Read the model definition and answer for the solid it produces. Units are mm, in the model's axes. A direction names the side the tool comes from. Give positions to 0.01 mm unless a question says otherwise; leave off trailing zeros. Write each loop counter-clockwise with the first axis right and the second up, starting at its lowest first coordinate (ties: lowest second). Pieces come first, ordered by that corner, then holes. Notation, with made-up numbers: M -20,-30 L -4,-30 A15 cw -4,-14 Z; hole C 51,-10 d6. An arc over 180 degrees is marked long. Use a Markdown table: item, result. Add a question column.
Item 1: The mould has two halves that part along X. Classify faces 1 (the flat face through (60, -77.788, 0)), 2 (the flat face through (-69.85, -109, 0)), 3 (the cylindrical face through (-37.26, -0.72, 9.57)): pulls with the +X half, pulls with the -X half, needs draft (parallel to the pull), parting line crosses it, or undercut.
Item 2: For faces 4 (the cylindrical face through (0.943, 42.852, 0.178)), 5 (the flat face through (0, 28, 6.35)), 6 (the flat face through (-42.862, -35, 0)), 7 (the cylindrical face through (0.73, 28.45, 0.55)), 8 (the cylindrical face through (31.201, -103.976, -9.569)), determine the directions among +Z, -Z, +X, -X, +Y, -Y from which every point of the face is accessible in a straight line to the end or side of a thin tool.
Item 3: A cutting plane is placed at C-C on x = 0. Count the separate pieces of the cut face and the enclosed holes in it, then the cut area to 3 significant figures.
Item 4: Given P1, Ø8, axis at y = -21.5, z = -3, coming from the +X side; P2, Ø4.5, axis at x = 22.5, y = -76.5, coming from the +Z side; P3, Ø5, axis at x = 36.5, z = 1, coming from the +Y side, each flat-ended and moving along its own axis, determine where each tip first touches the part or whether it passes through.
Item 5: A cutting plane is placed at A-A on x = -57.15. Determine the outline of the cut face in (y, z), then the cut area to 3 significant figures.
Item 6: Consider probe 1 along X at (y, z) = (0, 3); probe 2 along X at (y, z) = (0, 9.75); probe 3 along X at (y, z) = (-31.75, -2.25). Determine where each line is inside the solid, lowest interval first. Write a range as [from, to].
Item 7: A cutting plane is placed at B-B on y = -7.5. Determine the outline of the cut face in (x, z).
from build123d import *

# Parameters (mm, degrees)
BOLT_CIRCLE_R                                     = 12.7
BOLT_CIRCLE_R_2                                   = 6.35
BASE_DEPTH                                        = 12.7
STRUCTURE_TUBE_CONNECTION_COUNTERBORE_D           = 6.7564
STRUCTURE_TUBE_CONNECTION_COUNTERBORE_CBORE_D     = 11.1125
STRUCTURE_TUBE_CONNECTION_COUNTERBORE_CBORE_DEPTH = 6.35
STRUCTURE_TUBE_CONNECTION_COUNTERBORE_PA_COUNT    = 4
SPINDLE_CONNECTION_COUNTERBORE_D                  = 6.7564
SPINDLE_CONNECTION_COUNTERBORE_CBORE_D            = 11.1125
SPINDLE_CONNECTION_COUNTERBORE_CBORE_DEPTH        = 6.35
SPINDLE_CONNECTION_COUNTERBORE_PATTERN_COUNT      = 4
SKETCH16_R                                        = 36.5125
STRUCTURE_TUBE_MOUNTING_POCKET_DEPTH              = 6.35
SKETCH17_R                                        = 36.5125
SPINDLE_MOUNTING_POCKET_DEPTH                     = 7.62
SKETCH18_R                                        = 9.525
LEAD_SCREW_THROUGH_HOLE_DEPTH                     = 9.525
SKETCH20_R                                        = 7.9375
RAIL_MOUNTING_PILOT_HOLES_DEPTH                   = 166.290695159
SKETCH27_R                                        = 2.38125
ALIGNMENT_FEATURES_DEPTH                          = 6.35
GENERIC_ROUNDING_FILLET_R                         = 6.35


with BuildPart() as part:
    # Bolt circle → Base (new, symmetric)
    with BuildSketch(Plane.XY):
        with BuildLine():
            Line((-42.8625, 0), (-42.8625, -77.7875))
            Line((-42.8625, -77.7875), (-69.85, -77.7875))
            Line((-69.85, -77.7875), (-69.85, -147.6375))
            Line((-69.85, -147.6375), (69.85, -147.6375))
            Line((69.85, -147.6375), (69.85, -77.7875))
            Line((69.85, -77.7875), (42.8625, -77.7875))
            Line((42.8625, -77.7875), (42.8625, 0))
            ThreePointArc((42.8625, 0), (0, 42.8625), (-42.8625, 0))
        make_face()
        Circle(BOLT_CIRCLE_R, mode=Mode.SUBTRACT)
        with Locations((0, -98.425)):
            Circle(BOLT_CIRCLE_R_2, mode=Mode.SUBTRACT)
    extrude(amount=BASE_DEPTH, both=True)

    # Structure tube connection counterbore (through all)
    with Locations(Plane(origin=(0, 0, -12.7), x_dir=(-1, 0, 0), z_dir=(0, 0, -1))):
        with Locations((0, -67.46875)):
            structure_tube_connection_counterbore = CounterBoreHole(STRUCTURE_TUBE_CONNECTION_COUNTERBORE_D / 2, STRUCTURE_TUBE_CONNECTION_COUNTERBORE_CBORE_D / 2, STRUCTURE_TUBE_CONNECTION_COUNTERBORE_CBORE_DEPTH)

    # Structure tube connection counterbore pa: Structure tube connection counterbore ×4 about axis
    structure_tube_connection_counterbore_pa_axis = Axis((0, -98.425, 0), (0, 0, 1))
    for i in range(1, STRUCTURE_TUBE_CONNECTION_COUNTERBORE_PA_COUNT):
        add(structure_tube_connection_counterbore.rotate(structure_tube_connection_counterbore_pa_axis, i * 360 / STRUCTURE_TUBE_CONNECTION_COUNTERBORE_PA_COUNT), mode=Mode.SUBTRACT)

    # Spindle connection counterbore (through all)
    with Locations(Plane.XY.offset(12.7)):
        with Locations((0, 31.75)):
            spindle_connection_counterbore = CounterBoreHole(SPINDLE_CONNECTION_COUNTERBORE_D / 2, SPINDLE_CONNECTION_COUNTERBORE_CBORE_D / 2, SPINDLE_CONNECTION_COUNTERBORE_CBORE_DEPTH)

    # Spindle connection counterbore pattern: Spindle connection counterbore ×4 about axis
    spindle_connection_counterbore_pattern_axis = Axis((0, 0, 0), (0, 0, 1))
    for i in range(1, SPINDLE_CONNECTION_COUNTERBORE_PATTERN_COUNT):
        add(spindle_connection_counterbore.rotate(spindle_connection_counterbore_pattern_axis, i * 360 / SPINDLE_CONNECTION_COUNTERBORE_PATTERN_COUNT), mode=Mode.SUBTRACT)

    # Sketch16 → Structure tube mounting pocket (cut)
    with BuildSketch(Plane.XY.offset(12.7)):
        with Locations((0, -98.425)):
            Circle(SKETCH16_R)
    extrude(amount=-STRUCTURE_TUBE_MOUNTING_POCKET_DEPTH, mode=Mode.SUBTRACT)

    # Sketch17 → Spindle mounting pocket (cut)
    with BuildSketch(Plane(origin=(0, 0, -12.7), x_dir=(-1, 0, 0), z_dir=(0, 0, -1))):
        Circle(SKETCH17_R)
    extrude(amount=-SPINDLE_MOUNTING_POCKET_DEPTH, mode=Mode.SUBTRACT)

    # Sketch18 → Lead screw through hole (cut)
    with BuildSketch(Plane.XY.offset(6.35)):
        with Locations((0, -98.425)):
            Circle(SKETCH18_R)
    extrude(amount=-LEAD_SCREW_THROUGH_HOLE_DEPTH, mode=Mode.SUBTRACT)

    # Sketch20 → Rail mounting pilot_holes (cut, through all)
    with BuildSketch(Plane.XY.offset(12.7)):
        with Locations((57.15, -98.425)):
            Circle(SKETCH20_R)
        with Locations((-57.15, -98.425)):
            Circle(SKETCH20_R)
    extrude(amount=-RAIL_MOUNTING_PILOT_HOLES_DEPTH, mode=Mode.SUBTRACT)

    # Sketch27 → Alignment_features (cut)
    with BuildSketch(Plane.XY.offset(6.35)):
        with Locations((-21.889374295, -120.314374295)):
            Circle(SKETCH27_R)
        with BuildLine():
            Line((20.681324246, -74.335397148), (19.602797121, -75.500272889))
            ThreePointArc((19.602797121, -75.500272889), (19.732320046, -78.865377187), (23.097424344, -78.735854262))
            Line((23.097424344, -78.735854262), (24.175951469, -77.570978521))
            ThreePointArc((24.175951469, -77.570978521), (24.046428544, -74.205874223), (20.681324246, -74.335397148))
        make_face()
    extrude(amount=-ALIGNMENT_FEATURES_DEPTH, mode=Mode.SUBTRACT)

    # Generic_rounding_fillet
    generic_rounding_fillet_edges = [part.edges().sort_by_distance(p)[0] for p in [
        (-42.8625, -77.7875, 0),
        (42.8625, -77.7875, 0),
        (69.85, -147.6375, 0),
        (-69.85, -147.6375, 0),
    ]]
    fillet(generic_rounding_fillet_edges, radius=GENERIC_ROUNDING_FILLET_R)


solid = part.part
Filled in:
| question | item | result |
|---|---|---|
| 1 | face 1 | needs draft |
| 1 | face 2 | pulls with the -X half |
| 1 | face 3 | undercut |
| 2 | face 4 | +Z, -Z, +Y |
| 2 | face 5 | +Z |
| 2 | face 6 | +Z, -Z, -X, +Y |
| 2 | face 7 | +Z, -Z |
| 2 | face 8 | -Z |
| 3 | separate pieces | 7 |
| 3 | enclosed holes | 0 |
| 3 | area | 2,460 mm² |
| 4 | P1 | x = 42.86 |
| 4 | P2 | z = 6.35 |
| 4 | P3 | y = 26.1 |
| 5 | outline | M -147.64,-12.7 L -106.36,-12.7 L -106.36,12.7 L -147.64,12.7 Z; M -90.49,-12.7 L -77.79,-12.7 L -77.79,12.7 L -90.49,12.7 Z |
| 5 | area | 1,370 mm² |
| 6 | probe 1 | [-42.86, -35.13], [-28.37, -12.7], [12.7, 28.37], [35.13, 42.86] |
| 6 | probe 2 | [-42.86, -37.31], [-26.19, -12.7], [12.7, 26.19], [37.31, 42.86] |
| 6 | probe 3 | [-42.86, -3.38], [3.38, 42.86] |
| 7 | outline | M -42.86,-12.7 L -35.73,-12.7 L -35.73,-5.08 L -10.25,-5.08 L -10.25,12.7 L -42.86,12.7 Z; M 10.25,-5.08 L 35.73,-5.08 L 35.73,-12.7 L 42.86,-12.7 L 42.86,12.7 L 10.25,12.7 Z |
